Part model, mm, in its own coordinate system. Round coordinates to 2 decimals unless told otherwise and drop trailing zeros. Answer as a JSON object with one key per item and string values. Group by question number.
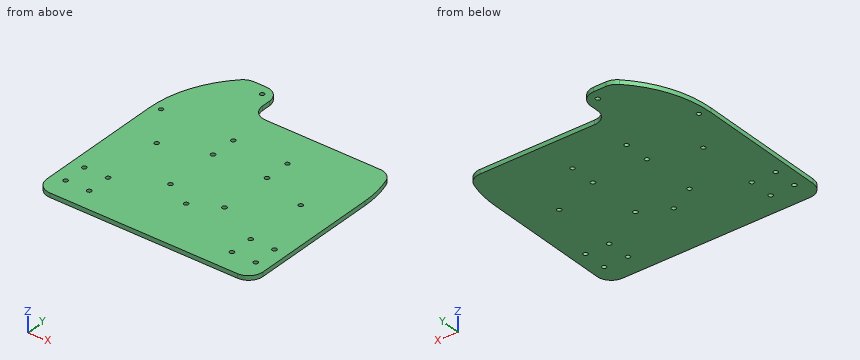
Autodesk Fusion 360 part; units mm, degrees
sketch "Sketch1" plane through (0, 0, 0) normal (0, 0, 1) x (1, 0, 0)
  circle A0 centre (0, 0) radius 75
  line L0 (-75, 0) -> (75, 0)
  line L1 (75, 0) -> (75, -100)
  line L2 (75, -100) -> (-75, -100)
  line L3 (-75, -100) -> (-75, 0)
  circle A1 centre (49.5, -68.5) radius 1.55
  circle A2 centre (66, -85) radius 1.55
  circle A3 centre (66, -68.5) radius 1.55
  circle A4 centre (49.5, -85) radius 1.55
  circle A5 centre (-66, -68.5) radius 1.55
  circle A6 centre (-66, -85) radius 1.55
  circle A7 centre (-49.5, -68.5) radius 1.55
  circle A8 centre (-49.5, -85) radius 1.55
  line L4 (-50, 55.9017) -> (50, 55.9017)
  circle A9 centre (-18.75, -52.5) radius 1.55
  circle A10 centre (18.75, -52.5) radius 1.55
  circle A11 centre (18.75, -15) radius 1.55
  circle A12 centre (-18.75, -15) radius 1.55
  line L5 (-69, 49) -> (-35, 49)
  line L6 (-35, 49) -> (-35, 3)
  line L7 (-35, 3) -> (-69, 3)
  line L8 (-69, 3) -> (-69, 49)
  circle A13 centre (-69, 3) radius 1.5
  circle A14 centre (-35, 49) radius 1.5
  circle A15 centre (-35, 49) radius 3
  circle A16 centre (-69, 3) radius 3
  line L9 (-27.5, 69.7764) -> (-27.5, 29.7764)
  line L10 (-27.5, 29.7764) -> (68.8358, 29.7764)
  circle A17 centre (-18.75, 3) radius 1.5
  circle A18 centre (18.75, 3) radius 1.5
  circle A19 centre (-50, -25) radius 1.5
  circle A20 centre (50, -25) radius 1.5
  circle A21 centre (0, -62.5) radius 1.5
  dimension "d1" = 150
  dimension "d2" = 150
  dimension "d3" = 100
  dimension "d4" = 3.1
  dimension "d5" = 3.1
  dimension "d6" = 3.1
  dimension "d7" = 3.1
  dimension "d8" = 3.1
  dimension "d9" = 3.1
  dimension "d10" = 3.1
  dimension "d11" = 3.1
  dimension "d12" = 16.5
  dimension "d14" = 16.5
  dimension "d15" = 16.5
  dimension "d16" = 16.5
  dimension "d17" = 16.5
  dimension "d18" = 16.5
  dimension "d20" = 16.5
  dimension "d21" = 16.5
  dimension "d22" = 9
  dimension "d23" = 9
  dimension "d24" = 15
  dimension "d25" = 15
  dimension "d26" = 100
  dimension "d27" = 3.1
  dimension "d28" = 3.1
  dimension "d29" = 3.1
  dimension "d30" = 3.1
  dimension "d36" = 37.5
  dimension "d37" = 37.5
  dimension "d38" = 37.5
  dimension "d39" = 37.5
  dimension "d46" = 15
  dimension "d47" = 18.75
  dimension "d55" = 34
  dimension "d56" = 46
  dimension "d57" = 3
  dimension "d58" = 40
  dimension "d59" = 3
  dimension "d60" = 3
  dimension "d73" = 6
  dimension "d74" = 6
  dimension "d86" = 40
  dimension "d87" = 7.5
  dimension "d88" = 3
  dimension "d89" = 3
  dimension "d90" = 37.5
  dimension "d91" = 18.75
  dimension "d92" = 3
  dimension "d95" = 3
  dimension "d96" = 3
  dimension "d97" = 100
  dimension "d98" = 50
  dimension "d99" = 25
  dimension "d100" = 3
  dimension "d101" = 18.75
  dimension "d102" = 10
extrude "Extrude7" add sketch "Sketch1" along normal blind 3 contours A0 L0 L4 L5 L6 L7 A15 A16 L9 L10 | A0 L1 L2 L3 | A0 L0 | A0 L0 L8 A16 | L7 L8 A13 A16 | A0 L5 L6 L7 L8 A15 A16 | L7 L8 A13 A16 | L5 L6 A14 A15 | L5 L6 A14 A15
fillet "Fillet6" radius 10 6 edges at (-27.5, 55.9017, 1.5) (75, -100, 1.5) (-75, -100, 1.5) (-50, 55.9017, 1.5) (68.8358, 29.7764, 1.5) (-27.5, 29.7764, 1.5)
Q1. Band-saw the part on A-A (z = 2.05). Count the separate pieces of the cut face and the enclosed holes in it, plus the area to 3 significant figures.
Q2. Wall check: line 1 (X direction, y = -68.5, z = 2.1); line 2 (Y direction, x = 50, z = 0.6); line 3 (X direction, y = -14, z = 1). Give the ranges that are in metal, low to high. Write a range as [from, to].
Q3. Drop flat-ended pins along their axis: pin 1 Ø1.5 at (y, z) = (42, 1.5) entering from +X; pin 2 Ø1.5 at (x, z) = (25.5, 0.5) entering from +Y. Give the stop position or say it passes through.
Completed:
{
 "1": {"separate pieces": "1", "enclosed holes": "19", "area": "20,000 mm2"},
 "2": {"line 1": "[-75, -67.55], [-64.45, -51.05], [-47.95, 47.95], [51.05, 64.45], [67.55, 75]", "line 2": "[-100, -86.47], [-83.53, -69.97], [-67.03, -26.5], [-23.5, 29.78]", "line 3": "[-75, -19.93], [-17.57, 17.57], [19.93, 75]"},
 "3": {"pin 1": "x = -27.5", "pin 2": "y = 29.78"}
}
